Here's how the part is built. I have some questions about the finished solid (model axes, mm). Face numbers are marked on the shaded views. Coordinates: 2 decimals unless noted, no trailing zeros. Write each loop counter-clockwise with the first axis right and the second up, starting at its lowest first coordinate (ties: lowest second). Pieces come first, ordered by that corner, then holes. Notation, with made-up numbers: (-31, -35) - (-25, -35) arc R18 ccw to (-25, -1) - close; hole circle Ø10 at (-15, 19.5). An arc over 180 degrees is marked (long way). Answer in a Markdown table with one row per item. Add a question column.
Item 1: I'm going to push flat-ended pins straight in: pin 1 (24 mm diameter, centred on x = -10.5, y = -56.5, fed in from -Z); pin 2 (4 mm diameter, centred on y = -7.5, z = 7, fed in from +X); pin 3 (13.5 mm diameter, centred on y = -37, z = 6, fed in from +X). Where does each tip first touch, or does it pass through?
Item 2: Imagine slicing it at C-C (y = -41). Please give me the cut outline in (x, z), plus the area to 3 significant figures.
Item 3: If I drill on probe 1 along Y at (x, z) = (0, 18); probe 2 along Y at (x, z) = (-42.5, -21.5); probe 3 along X at (y, z) = (-3, -39), over which ranges is the centre line in solid material (lowest first)? Write a range as from..to.
Item 4: Imagine slicing it at D-D (y = -11). Please give me the cut outline in (x, z), plus the area to 3 significant figures.
Item 5: Imagine slicing it at A-A (x = 0). Please give me the cut outline in (y, z), plus the area to 3 significant figures.
Item 6: Imagine slicing it at B-B (z = -29). Please give me the cut outline in (x, y), plus the area to 3 significant figures.
Item 7: We'd pull the mould along X, two halves only. Please class the marked faces 1, 2, 3 and 4: +X half, -X half, draft (parallel to the pull), parting line (faces both ways), or undercut.
from build123d import *

# Parameters (mm, degrees)
F0_R     = 10
F1_DEPTH = 15
F3_R     = 15
F4_DEPTH = 15
F5_R     = 12


# Not quite as in the source:
# - ends of sketch curves that miss each other by under 0.0002 mm in the source are joined


with BuildPart() as f1:
    # F0 (on Front) → F1 (new body)
    with BuildSketch(Plane.XZ):
        with BuildLine():
            Line((-30, 24.9995148627), (-69.9428552721, -27.4248908346))
            ThreePointArc((-69.9428552721, -27.4248908346), (-71.2014492094, -40.5482356371), (-60, -47.5004851373))
            Line((-60, -47.5004851373), (60, -47.5004851373))
            ThreePointArc((60, -47.5004851373), (71.2014492094, -40.5482356371), (69.9428552721, -27.4248908346))
            Line((69.9428552721, -27.4248908346), (30, 24.9995148627))
            Line((30, 24.9995148627), (0, 24.9995148627))
            Line((0, 24.9995148627), (-30, 24.9995148627))
        make_face()
        with Locations((-60, -35.0004851373)):
            Circle(F0_R, mode=Mode.SUBTRACT)
        with Locations((60, -35.0004851373)):
            Circle(F0_R, mode=Mode.SUBTRACT)
    extrude(amount=F1_DEPTH)

    # F3 (on offset) → F4 (join)
    with BuildSketch(Plane.XY.offset(24.9995148627)):
        with BuildLine():
            Line((-30, -14.9999307469), (-30, -45.0000600332))
            ThreePointArc((-30, -45.0000600332), (2.21189e-05, -75), (30, -45.0000157953))
            Line((30, -45.0000157953), (30, -14.9999307469))
            Line((30, -14.9999307469), (30, 0))
            Line((30, 0), (-30, 0))
            Line((-30, 0), (-30, -14.9999307469))
        make_face()
        with Locations((0, -45)):
            Circle(F3_R, mode=Mode.SUBTRACT)
    extrude(amount=-F4_DEPTH)

    # F5
    f5_edges = [f1.edges().sort_by_distance(p)[0] for p in [
        (0, -15, 9.999515),
    ]]
    fillet(f5_edges, radius=F5_R)


solid = f1.part
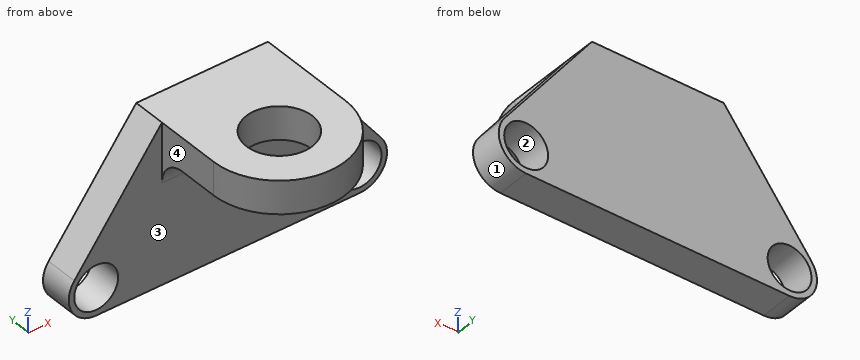
Here are the results:
| question | item | result |
|---|---|---|
| 1 | pin 1 | stops at z = 10 |
| 1 | pin 2 | stops at x = 45.24 |
| 1 | pin 3 | stops at x = 30 |
| 2 | outline | (-30, 10) - (-14.46, 10) - (-14.46, 25) - (-30, 25) - close; (14.46, 10) - (30, 10) - (30, 25) - (14.46, 25) - close |
| 2 | area | 466 mm2 |
| 3 | probe 1 | y = -75..-60, -30..0 |
| 3 | probe 2 | y = -15..0 |
| 3 | probe 3 | x = -71.84..-69.17, -50.83..50.83, 69.17..71.84 |
| 4 | outline | (-69.94, -27.42) arc R12.5 ccw to (-60, -47.5) - (60, -47.5) arc R12.5 ccw to (69.94, -27.42) - (30, 25) - (-30, 25) - close; hole circle Ø20 at (-60, -35); hole circle Ø20 at (60, -35) |
| 4 | area | 7,440 mm2 |
| 5 | outline | (-75, 10) - (-60, 10) - (-60, 25) - (-75, 25) - close; (-30, 10) - (-27, 10) arc R12 cw to (-15, -2) - (-15, -47.5) - (0, -47.5) - (0, 25) - (-30, 25) - close |
| 5 | area | 1,570 mm2 |
| 6 | outline | (-70.97, -15) - (-68, -15) - (-68, 0) - (-70.97, 0) - close; (-52, -15) - (52, -15) - (52, 0) - (-52, 0) - close; (68, -15) - (70.97, -15) - (70.97, 0) - (68, 0) - close |
| 6 | area | 1,650 mm2 |
| 7 | face 1 | +X half |
| 7 | face 2 | undercut |
| 7 | face 3 | draft |
| 7 | face 4 | -X half |
